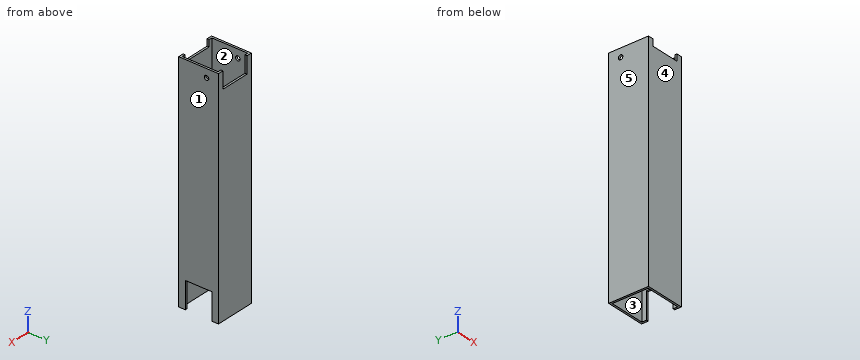
from build123d import *

# Parameters (mm, degrees)
F0_W     = 60
F0_H     = 60
F0_W_2   = 54
F0_H_2   = 54
F1_DEPTH = 340
F2_W     = 40
F2_H     = 40
F3_DEPTH = 3
F4_W     = 44
F4_H     = 25
F5_DEPTH = 3
F7_D     = 6.8
F8_W     = 44
F8_H     = 10
F9_DEPTH = 25


with BuildPart() as f1:
    # F0 (on Top) → F1 (new body)
    with BuildSketch(Plane.XY):
        with Locations((30, 30)):
            Rectangle(F0_W, F0_H)
        with Locations((30, 30)):
            Rectangle(F0_W_2, F0_H_2, mode=Mode.SUBTRACT)
    extrude(amount=F1_DEPTH)

    # F2 (on face) → F3 (cut)
    with BuildSketch(Plane.YZ.offset(60)):
        with Locations((30, 20)):
            Rectangle(F2_W, F2_H)
    extrude(amount=-F3_DEPTH, mode=Mode.SUBTRACT)

    # F4 (on face) → F5 (cut)
    with BuildSketch(Plane(origin=(0, 60, 0), x_dir=(-1, 0, 0), z_dir=(0, 1, 0))):
        with Locations((-30, 327.5)):
            Rectangle(F4_W, F4_H)
    extrude(amount=-F5_DEPTH, mode=Mode.SUBTRACT)

    # F7 (through all)
    with Locations(Plane.YZ.offset(60)):
        with Locations((42, 327.3)):
            Hole(F7_D / 2)

    # F8 (on face) → F9 (cut)
    with BuildSketch(Plane.XZ):
        with Locations((30, 335)):
            Rectangle(F8_W, F8_H)
    extrude(amount=-F9_DEPTH, mode=Mode.SUBTRACT)


solid = f1.part
Here's how the part is built. I have some questions about the finished solid (model axes, mm). Face numbers are marked on the shaded views. A direction names the side the tool comes from. Round coordinates to 2 decimals unless told otherwise and drop trailing zeros. Loops run counter-clockwise (first coordinate to the right, second up) from the corner with the lowest first, then second, coordinate; pieces in that order, holes last. Notation, with made-up numbers: M 78.5,5.25 L 83.5,5.25 A24 ccw 83.5,23.25 Z; hole C 88.5,77.5 d1. An arc over 180 degrees is marked long. Write each question's results on one line, items separated by ' | '. Start each with the question number.
(1) If I drill on probe 1 along X at (y, z) = (54.5, 137.5); probe 2 along Y at (x, z) = (58, 327), over which ranges is the centre line in solid material (lowest first)? Write a range as from..to.
(2) Will these pins go through, and if not, where does the flat tip stop? P1, Ø2.5, axis at x = 26.5, y = 58.5, coming from the +Z side; P2, Ø3.5, axis at x = 59, y = 35.5, coming from the -Z side; P3, Ø2.5, axis at x = 25, y = 1.5, coming from the +Z side.
(3) On a 3-axis mill with a long thin cutter (end or side, diameter ignored), from which of +Z, -Z, +X, -X, +Y, -Y can I reach the whole of each face in a straight line? I mean the marked faces 1 and 2. Say none if no direction works.
(4) I want a section at C-C (y = 20). Please give me the cut outline in (x, z).
(5) I want a section at A-A (y = 42). Please give me the cut outline in (x, z), then the cut area to 3 significant figures.
(6) Thinking about a two-plate mould opening in X: for the marked faces 3, 4 and 5, which applies, pulls with the +X half, pulls with the -X half, needs draft (parallel to the pull), parting line crosses it, or undercut?
(7) I want a section at D-D (z = 165.5). Please give me the cut outline in (x, y).
(8) I want a section at B-B (x = 36). Please give me the cut outline in (y, z).
Solved:
1) probe 1: x = 0..3, 57..60 | probe 2: y = 0..38.61, 45.39..60
2) P1: stops at z = 315 | P2: stops at z = 40 | P3: stops at z = 330
3) face 1: +Z, -Z, +X, +Y, -Y | face 2: +Z, -Z
4) outline: M 0,0 L 3,0 L 3,340 L 0,340 Z; M 57,40 L 60,40 L 60,340 L 57,340 Z
5) outline: M 0,0 L 3,0 L 3,323.9 L 0,323.9 Z; M 0,330.7 L 3,330.7 L 3,340 L 0,340 Z; M 57,40 L 60,40 L 60,323.9 L 57,323.9 Z; M 57,330.7 L 60,330.7 L 60,340 L 57,340 Z | area: 1,880 mm²
6) face 3: undercut | face 4: needs draft | face 5: pulls with the -X half
7) outline: M 0,0 L 60,0 L 60,60 L 0,60 Z; hole M 3,3 L 57,3 L 57,57 L 3,57 Z
8) outline: M 0,0 L 3,0 L 3,330 L 0,330 Z; M 57,0 L 60,0 L 60,315 L 57,315 Z
